from build123d import *

# Parameters (mm, degrees)
F0_W     = 88.9
F0_H     = 44.45
F1_DEPTH = 12.7
F2_R     = 9.525
F4_DEPTH = 12.7
F5_R     = 19.05
F5_R_2   = 9.525
F6_DEPTH = 44.45
F7_R     = 9.525
F8_DEPTH = 44.45
F9_R     = 6.35


with BuildPart() as f1:
    # F0 (on Front) → F1 (new body)
    with BuildSketch(Plane.XZ):
        with Locations((44.45, -13.911705)):
            Rectangle(F0_W, F0_H)
    extrude(amount=F1_DEPTH)

    # F2
    f2_edges = [f1.edges().sort_by_distance(p)[0] for p in [
        (88.9, -6.35, 8.313295),
        (88.9, -6.35, -36.136705),
    ]]
    fillet(f2_edges, radius=F2_R)

    # F3 (on face) → F4 (cut)
    with BuildSketch(Plane.XZ.offset(12.7)):
        with BuildLine():
            ThreePointArc((38.1, -21.849205), (43.71266, -19.524366), (46.0375, -13.911705))
            ThreePointArc((46.0375, -13.911705), (43.71266, -8.299045), (38.1, -5.974205))
            ThreePointArc((38.1, -5.974205), (30.1625, -13.911705), (38.1, -21.849205))
        make_face()
        with BuildLine():
            ThreePointArc((38.1, -5.974205), (43.71266, -8.299045), (46.0375, -13.911705))
            ThreePointArc((46.0375, -13.911705), (43.71266, -19.524366), (38.1, -21.849205))
            Line((38.1, -21.849205), (88.9, -21.849205))
            Line((88.9, -21.849205), (88.9, -5.974205))
            Line((88.9, -5.974205), (38.1, -5.974205))
        make_face()
    extrude(amount=-F4_DEPTH, mode=Mode.SUBTRACT)

    # F5 (on face) → F6 (join)
    with BuildSketch(Plane.XY.offset(8.313295)):
        with Locations((0, -19.242762)):
            Circle(F5_R)
        with Locations((0, -19.242762)):
            Circle(F5_R_2, mode=Mode.SUBTRACT)
    extrude(amount=-F6_DEPTH)

    # F7 (on face) → F8 (cut)
    with BuildSketch(Plane.XY.offset(8.313295)):
        with Locations((0, -19.242762)):
            Circle(F7_R)
    extrude(amount=-F8_DEPTH, mode=Mode.SUBTRACT)

    # F9
    f9_edges = [f1.edges().sort_by_distance(p)[0] for p in [
        (17.891192, -12.7, -13.911705),
    ]]
    fillet(f9_edges, radius=F9_R)


solid = f1.part
CAD build for the part. Positions are in the model's coordinates, mm. A direction names the side the tool comes from. Coordinates: 2 decimals unless noted, no trailing zeros. Write each loop counter-clockwise with the first axis right and the second up, starting at its lowest first coordinate (ties: lowest second). Pieces come first, ordered by that corner, then holes. Notation, with made-up numbers: M 37.5,-31.75 L 66.5,-31.75 A19 cw 66.5,-20.75 Z; hole C 50,-26.75 d4. An arc over 180 degrees is marked long. Answer as a JSON object with one key per item and string values. Group by question number.
1) Pin check, flat tips, straight feed: pin 1 Ø13.5 at (x, z) = (68, -17) entering from -Y; pin 2 Ø5 at (y, z) = (-30, -25) entering from -X; pin 3 Ø17 at (x, y) = (0, -19.24) entering from +Z; pin 4 Ø3 at (y, z) = (-15, -0.5) entering from -X. Stop position of each tip, or through.
2) Saw through at B-B (y = -27.5). Write the cut outline in (x, z), plus the area to 3 significant figures.
3) Saw through at D-D (z = -12). Write the cut outline in (x, y) (3 decimals), plus the area to 3 significant figures.
4) Saw through at C-C (z = 0). Write the cut outline in (x, y) (3 decimals), plus the area to 3 significant figures.
5) Saw through at A-A (x = 54). Write the cut outline in (y, z), plus the area to 3 significant figures.
6) Wall check: line 1 (Z direction, x = 79, y = -10.5); line 2 (X direction, y = -19.5, z = -31.5); line 3 (Y direction, x = 67, z = -25.5). Give the ranges that are in metal, low to high. Write a range as from..to.
7) Tool access for faces 1 (the face through (-1.512, -28.647, -13.601)), 2 (the face through (64, -6, -5.974)), 3 (the face through (57, -12.7, -23)): list every direction of +Z, -Z, +X, -X, +Y, -Y with a clear straight run to the whole face (end or side of a thin tool).
8) Mould opens along Z. For faces 4 (the face through (86.036, -6.439, -33.421)), 5 (the face through (20.84, -14.63, -13.6)), 6 (the face through (63, -6, -21.849)) say: +Z half, -Z half, draft (parallel to the pull), parting line (faces both ways), or undercut.
Values follow:
{
 "1": {"pin 1": "stops at y = -12.7", "pin 2": "stops at x = -17.17", "pin 3": "passes through", "pin 4": "stops at x = -18.85"},
 "2": {"outline": "M -17.17,-36.14 L -4.75,-36.14 L -4.75,8.31 L -17.17,8.31 Z; M 4.75,-36.14 L 17.17,-36.14 L 17.17,8.31 L 4.75,8.31 Z", "area": "1,100 mm2"},
 "3": {"outline": "M 0,-0.193 A19.05 ccw long 19.049,-19.098 A6.35 cw 25.399,-12.7 L 30.396,-12.7 L 30.396,0 L 0,0 Z; hole C 0,-19.243 d19.05", "area": "1,090 mm2"},
 "4": {"outline": "M 0,-0.193 A19.05 ccw long 19.049,-19.098 A6.35 cw 25.399,-12.7 L 88.823,-12.7 L 88.823,0 L 0,0 Z; hole C 0,-19.243 d19.05", "area": "1,830 mm2"},
 "5": {"outline": "M -12.7,-36.14 L 0,-36.14 L 0,-21.85 L -12.7,-21.85 Z; M -12.7,-5.97 L 0,-5.97 L 0,8.31 L -12.7,8.31 Z", "area": "363 mm2"},
 "6": {"line 1": "z = -36.14..-21.85, -5.97..8.31", "line 2": "x = -19.05..-9.52, 9.52..19.05", "line 3": "y = -12.7..0"},
 "7": {"face 1": "+Z, -Z", "face 2": "+X, +Y, -Y", "face 3": "+Z, -Z, +X, -Y"},
 "8": {"face 4": "-Z half", "face 5": "draft", "face 6": "undercut"}
}
